```python
from build123d import *

# Parameters (mm, degrees)
BOSS_EXTRUDE1_DEPTH = 5
BOSS_EXTRUDE2_DEPTH = 7.5
SKETCH3_W           = 5
SKETCH3_H           = 35
BOSS_EXTRUDE3_DEPTH = 7.5
SKETCH4_W           = 5
SKETCH4_H           = 35
BOSS_EXTRUDE4_DEPTH = 5
BOSS_EXTRUDE5_DEPTH = 5
SKETCH7_R           = 1.8
CUT_EXTRUDE1_DEPTH  = 6


with BuildPart() as part:
    # Sketch1 → Boss-Extrude1 (new body)
    with BuildSketch(Plane.XY):
        Polygon((-7.529880478, -25.806772908), (27.470119522, -25.806772908), (27.470119522, -10.806772908), (7.470119522, -10.806772908), (7.470119522, 9.193227092), (-7.529880478, 9.193227092), align=None)
    extrude(amount=BOSS_EXTRUDE1_DEPTH)



with BuildPart() as body_2:
    # Sketch2 → Boss-Extrude2 (new body)
    with BuildSketch(Plane(origin=(0, 0, 0), x_dir=(-1, 0, 0), z_dir=(0, 0, -1))):
        Polygon((-7.470119522, 9.193227092), (-12.470119522, 9.193227092), (-12.470119522, -5.806772908), (-27.470119522, -5.806772908), (-27.470119522, -10.806772908), (-7.470119522, -10.806772908), align=None)
    extrude(amount=BOSS_EXTRUDE2_DEPTH)


with BuildPart() as body_3:
    # Sketch3 → Boss-Extrude3 (new body)
    with BuildSketch(Plane(origin=(0, 0, 0), x_dir=(-1, 0, 0), z_dir=(0, 0, -1))):
        with Locations((10.029880478, -8.306772908)):
            Rectangle(SKETCH3_W, SKETCH3_H)
    extrude(amount=BOSS_EXTRUDE3_DEPTH)


with BuildPart() as part_1:
    add(part.part)

    add(body_3.part)  # Boss-Extrude4 merges body 3
    # Sketch4 → Boss-Extrude4 (add)
    with BuildSketch(Plane.XY):
        with Locations((-10.029880478, -8.306772908)):
            Rectangle(SKETCH4_W, SKETCH4_H)
    extrude(amount=BOSS_EXTRUDE4_DEPTH)


    add(body_2.part)  # Boss-Extrude5 merges body 2
    # Sketch5 → Boss-Extrude5 (add)
    with BuildSketch(Plane.XY):
        Polygon((7.470119522, 9.193227092), (7.470119522, -10.806772908), (27.470119522, -10.806772908), (27.470119522, -5.806772908), (12.470119522, -5.806772908), (12.470119522, 9.193227092), align=None)
    extrude(amount=BOSS_EXTRUDE5_DEPTH)

    # Sketch7 → Cut-Extrude1 (cut, through all)
    with BuildSketch(Plane(origin=(0, 0, 0), x_dir=(-1, 0, 0), z_dir=(0, 0, -1))):
        with Locations((0.029880478, 1.693227092)):
            Circle(SKETCH7_R)
        with Locations((-17.470119522, -18.306772908)):
            Circle(SKETCH7_R)
    extrude(amount=-CUT_EXTRUDE1_DEPTH, mode=Mode.SUBTRACT)


solid = part_1.part
```
Work out the finished part from the listing and answer in its coordinate system (mm). A direction names the side the tool comes from. Coordinates: 2 decimals unless noted, no trailing zeros. Loops run counter-clockwise (first coordinate to the right, second up) from the corner with the lowest first, then second, coordinate; pieces in that order, holes last.
1) Consider probe 1 along Z at (x, y) = (7, 2); probe 2 along Y at (x, z) = (16.5, 3); probe 3 along X at (y, z) = (-7, -4.5). Determine where each line is inside the solid, lowest interval first.
Results:
probe 1: z = 0 to 5
probe 2: y = -25.81 to -19.82, -16.79 to -5.81
probe 3: x = -12.53 to -7.53, 7.47 to 27.47
2) Section C-C (x = 12) is taken. Give the vertices of the cut face in (y, z), plus the area to 3 significant figures.
Results:
outline: (-25.81, 0) - (-10.81, 0) - (-10.81, -7.5) - (9.19, -7.5) - (9.19, 5) - (-25.81, 5) - close
area: 325 mm2
3) Section A-A (z = -6) is taken. Give the vertices of the cut face in (x, y).
Results:
outline: (-12.53, -25.81) - (-7.53, -25.81) - (-7.53, 9.19) - (-12.53, 9.19) - close; (7.47, -10.81) - (27.47, -10.81) - (27.47, -5.81) - (12.47, -5.81) - (12.47, 9.19) - (7.47, 9.19) - close
4) For a pull along Y with two mould halves and no side action, classify faces 4 (the cylindrical face through (16.64, -19.904, 2.465)), 5 (the flat face through (12.47, 2, -1)), 6 (the flat face through (20, -5.807, -1)) as +Y half, -Y half, draft (parallel to the pull), parting line (faces both ways), or undercut.
Results:
face 4: undercut
face 5: draft
face 6: +Y half
5) Section D-D (x = 1) is taken. Give the vertices of the cut face in (y, z).
Results:
outline: (-25.81, 0) - (0.22, 0) - (0.22, 5) - (-25.81, 5) - close; (3.17, 0) - (9.19, 0) - (9.19, 5) - (3.17, 5) - close
6) Section B-B (y = -8) is taken. Give the vertices of the cut face in (x, z), plus the area to 4 significant figures.
Results:
outline: (-12.53, -7.5) - (-7.53, -7.5) - (-7.53, 0) - (7.47, 0) - (7.47, -7.5) - (27.47, -7.5) - (27.47, 5) - (-12.53, 5) - close
area: 387.5 mm2
7) For faces 1 (the flat face through (18, -10.807, -4)), 2 (the cylindrical face through (0.36, -0.064, 2.465)), 3 (the flat face through (7.47, -1, -4)), determine the directions among +Z, -Z, +X, -X, +Y, -Y from which every point of the face is accessible in a straight line to the end or side of a thin tool.
Results:
face 1: -Z, +X, -Y
face 2: +Z, -Z
face 3: -Z, +Y, -Y
8) Flat-ended cylindrical pins translate along their axes: pin 1 (6 mm diameter, centred on x = 17.47, y = -18.31, fed in from -Z); pin 2 (4 mm diameter, centred on y = -1.5, z = -2.5, fed in from +X); pin 3 (6 mm diameter, centred on x = 6.5, z = -1, fed in from -Y); pin 4 (6 mm diameter, centred on x = 22, z = -4, fed in from -Y). Find the tip coordinate at first contact, or state that the pin passes through.
Results:
pin 1: stops at z = 0
pin 2: stops at x = 12.47
pin 3: stops at y = -25.81
pin 4: stops at y = -10.81
